```python
from build123d import *

# Parameters (mm, degrees)
ESQUISSE1_W             = 180
ESQUISSE1_H             = 80
BOSS_EXTRU_1_DEPTH      = 4
ENL_V_MAT_EXTRU_1_DEPTH = 4
D_GAGEMENT_M22_D        = 2.4
D_GAGEMENT_M23_D        = 2.4


with BuildPart() as part:
    # Esquisse1 → Boss.-Extru.1 (new body)
    with BuildSketch(Plane(origin=(0, 0, 0), x_dir=(1, 0, 0), z_dir=(0, 1, 0))):
        with Locations((90, 40)):
            Rectangle(ESQUISSE1_W, ESQUISSE1_H)
    extrude(amount=BOSS_EXTRU_1_DEPTH)

    # Esquisse2 → Enlèv. mat.-Extru.1 (cut)
    with BuildSketch(Plane(origin=(0, 4, 0), x_dir=(1, 0, 0), z_dir=(0, 1, 0))):
        Polygon((0, 15), (30, 0), (0, 0), align=None)
        Polygon((30, 80), (0, 65), (0, 80), align=None)
        Polygon((150, 80), (180, 80), (180, 65), align=None)
        Polygon((180, 15), (150, 0), (180, 0), align=None)
    extrude(amount=-ENL_V_MAT_EXTRU_1_DEPTH, mode=Mode.SUBTRACT)

    # Dégagement M22 (through all)
    with Locations(Plane(origin=(0, 4, 0), x_dir=(1, 0, 0), z_dir=(0, 1, 0))):
        with Locations((74.75, 55.25), (105.25, 55.25), (105.25, 24.75), (74.75, 24.75)):
            Hole(D_GAGEMENT_M22_D / 2)

    # Dégagement M23 (through all)
    with Locations(Plane(origin=(0, 4, 0), x_dir=(1, 0, 0), z_dir=(0, 1, 0))):
        with Locations((34.75, 24.75), (65.25, 24.75), (65.25, 55.25), (34.75, 55.25)):
            Hole(D_GAGEMENT_M23_D / 2)


solid = part.part
```
Geometry check sheet. Reference: the model listing, model coordinates, mm. Give positions to 0.01 mm unless a question says otherwise; leave off trailing zeros. Write each loop counter-clockwise with the first axis right and the second up, starting at its lowest first coordinate (ties: lowest second). Pieces come first, ordered by that corner, then holes. Notation, with made-up numbers: (72.5, 32) -> (84.5, 32) arc R24 cw to (84.5, 68) -> close; hole circle Ø3 at (-24.5, -17). An arc over 180 degrees is marked (long way). Use one line per item in the form item = value.
Item 1: Depth check by flat-ended pin: pin 1 Ø1.4 at (x, z) = (34.75, -55.25) entering from +Y. Enter the tip coordinate at first touch or a pass-through.
Results list:
pin_1 = through
Item 2: Sectioned sample at B-B on z = -6. Enter the section's corners in (x, y).
Results list:
outline = (18, 0) -> (162, 0) -> (162, 4) -> (18, 4) -> close
Item 3: Scan lines: line 1 (X direction, y = 2.2, z = -55.25); line 2 (Z direction, x = 105.25, y = 2.65); line 3 (X direction, y = 2.7, z = -4). Record each from-to range of solid material in increasing order.
Results list:
line_1 = 0 to 33.55, 35.95 to 64.05, 66.45 to 73.55, 75.95 to 104.05, 106.45 to 180
line_2 = -80 to -56.45, -54.05 to -25.95, -23.55 to 0
line_3 = 22 to 158
Item 4: Sectioned sample at A-A on y = 1.6. Count the separate pieces of the cut face and the enclosed holes in it, plus the area to 3 significant figures.
Results list:
separate_pieces = 1
enclosed_holes = 8
area = 13,500 mm2
